```python
from build123d import *

# Parameters (mm, degrees)
F0_W     = 25
F0_H     = 25
F0_R     = 1.5
F3_DEPTH = 3
F4_R     = 5
F1_W     = 25
F1_H     = 25
F1_R     = 1.5
F5_DEPTH = 3
F6_R     = 5
F2_W     = 25
F2_H     = 25
F2_R     = 1.5
F7_DEPTH = 3
F8_R     = 5


with BuildPart() as f3:
    # F0 (on Top) → F3 (new body)
    with BuildSketch(Plane.XY):
        with Locations((-12.5, -12.5)):
            Rectangle(F0_W, F0_H)
        with Locations((-16, -16)):
            Circle(F0_R, mode=Mode.SUBTRACT)
    extrude(amount=F3_DEPTH)

    # F4
    f4_edges = [f3.edges().sort_by_distance(p)[0] for p in [
        (-25, -25, 1.5),
    ]]
    fillet(f4_edges, radius=F4_R)

    # F1 (on Right) → F5 (join)
    with BuildSketch(Plane.YZ):
        with Locations((-12.5, 12.5)):
            Rectangle(F1_W, F1_H)
        with Locations((-16, 16)):
            Circle(F1_R, mode=Mode.SUBTRACT)
    extrude(amount=F5_DEPTH)

    # F6
    f6_edges = [f3.edges().sort_by_distance(p)[0] for p in [
        (1.5, -25, 25),
    ]]
    fillet(f6_edges, radius=F6_R)

    # F2 (on Front) → F7 (join)
    with BuildSketch(Plane.XZ):
        with Locations((-12.5, 12.5)):
            Rectangle(F2_W, F2_H)
        with Locations((-16, 16)):
            Circle(F2_R, mode=Mode.SUBTRACT)
    extrude(amount=F7_DEPTH)

    # F8
    f8_edges = [f3.edges().sort_by_distance(p)[0] for p in [
        (-25, -1.5, 25),
    ]]
    fillet(f8_edges, radius=F8_R)


solid = f3.part
```
Geometry: final body of the model. Coordinates: model frame, mm. A direction names the side the tool comes from. Round coordinates to 2 decimals unless told otherwise and drop trailing zeros. Write each loop counter-clockwise with the first axis right and the second up, starting at its lowest first coordinate (ties: lowest second). Pieces come first, ordered by that corner, then holes. Notation, with made-up numbers: M 76,21.25 L 118,21.25 A21 ccw 118,51.25 Z; hole C 53.25,69.5 d1. An arc over 180 degrees is marked long. Answer in a Markdown table with one row per item. Add a question column.
(1) Contact query for flat-ended pins moving along their axis: pin 1 (11 mm diameter, centred on x = -17, z = 12.5, fed in from -Y); pin 2 (2.5 mm diameter, centred on y = -16, z = 16, fed in from +X); pin 3 (6.5 mm diameter, centred on y = -19.5, z = 19.5, fed in from -X). Output: stop coordinate, or through.
(2) Cut plane A-A, the plane y = -16. Return the cut outline in (x, z).
(3) Cut plane C-C, the plane z = 4.5. Return the cut outline in (x, y), then the cut area to 3 significant figures.
(4) Cut plane B-B, the plane x = -16. Return the cut outline in (y, z).
(5) Cut plane D-D, the plane x = -8.5. Return the cut outline in (y, z), then the cut area to 3 significant figures.
(6) Reachability of faces 1 (the face through (2, -24, 23)), 2 (the face through (-13, -14, 3)) from +Z, -Z, +X, -X, +Y, -Y: full face, straight path, thin tool, end or side. Return the list, or none.
(7) Draft query along Y for faces 3 (the face through (-13, -3, 14)), 4 (the face through (-17.5, -15.93, 1.48)), 5 (the face through (-4.3, -2.6, 25)). Return one class per face: pulls with the +Y half, pulls with the -Y half, needs draft (parallel to the pull), parting line crosses it, or undercut.
(8) Ray query, L1, parallel to Z at x = 2.3, y = -16; L2, parallel to Y at x = -16, z = 2; L3, parallel to Y at x = -9.75, z = 14.75. Return the intervals inside material, ascending.
Established:
| question | item | result |
|---|---|---|
| 1 | pin 1 | y = -3 |
| 1 | pin 2 | through |
| 1 | pin 3 | x = 0 |
| 2 | outline | M -25,0 L -17.5,0 L -17.5,3 L -25,3 Z; M -14.5,0 L 3,0 L 3,14.5 L 0,14.5 L 0,3 L -14.5,3 Z; M 0,17.5 L 3,17.5 L 3,25 L 0,25 Z |
| 3 | outline | M -25,-3 L 0,-3 L 0,-25 L 3,-25 L 3,0 L -25,0 Z |
| 3 | area | 150 mm² |
| 4 | outline | M -25,0 L -17.5,0 L -17.5,3 L -25,3 Z; M -14.5,0 L 0,0 L 0,14.5 L -3,14.5 L -3,3 L -14.5,3 Z; M -3,17.5 L 0,17.5 L 0,25 L -3,25 Z |
| 5 | outline | M -25,0 L 0,0 L 0,25 L -3,25 L -3,3 L -25,3 Z |
| 5 | area | 141 mm² |
| 6 | face 1 | +Z, +X, -X, -Y |
| 6 | face 2 | +Z, -X, -Y |
| 7 | face 3 | pulls with the -Y half |
| 7 | face 4 | undercut |
| 7 | face 5 | needs draft |
| 8 | L1 | 0 to 14.5, 17.5 to 25 |
| 8 | L2 | -25 to -17.5, -14.5 to 0 |
| 8 | L3 | -3 to 0 |
